Autodesk Inventor part; units mm, degrees
ref_plane "Arbeitsebene1" through (114.85, 0, 0) normal (1, 0, 0) x (0, 1, 0)
ref_plane "Arbeitsebene2" through (25.15, 0, 0) normal (1, 0, 0) x (0, 1, 0)
ref_plane "YZ Plane" through (0, 0, 0) normal (1, 0, 0) x (0, 1, 0)
sketch "Skizze1" plane through (0, 0, 0) normal (1, 0, 0) x (0, 1, 0)
  circle A0 centre (0, 0) radius 5
  dimension "d0" = 10
extrude "Extrusion1" add sketch "Skizze1" along normal blind 140
sketch "Skizze2" plane through (0, 0, 0) normal (-1, 0, 0) x (0, 0, 1)
  point P0 (0, 0)
  point P1 (0, 0)
hole "Bohrung1" at (0, 0, 0) direction (1, 0, 0) diameter 4.134 depth 14.2 tip angle 118
sketch "Skizze3" plane through (140, 0, 0) normal (1, 0, 0) x (0, 0, -1)
  point P0 (0, 0)
  point P1 (0, 0)
hole "Bohrung2" at (140, 0, 0) direction (-1, 0, 0) diameter 4.134 depth 14.2 tip angle 118
sketch "Skizze4" plane through (0, 0, 0) normal (0, 1, 0) x (-1, 0, 0)
  line L0 (0, 0) -> (-70, 0)
  line L1 (-70, 0) -> (-140, 0)
  line L2 (-140, -2.067) -> (-140, 2.067)
  line L3 (-70, 0) -> (-114.85, 0)
  line L4 (-70, 0) -> (-25.15, 0)
  dimension "d17" = 70
  dimension "d18" = 70
  dimension "d19" = 44.85
  dimension "d23" = 44.85
ref_plane "Arbeitsebene1" through (114.85, 0, 0) normal (1, 0, 0) x (0, 1, 0)
sketch "Skizze5" plane through (114.85, 0, 0) normal (1, 0, 0) x (0, 1, 0)
  circle A0 centre (0, 0) radius 5
  circle A1 centre (0, 0) radius 4
  dimension "d20" = 8
extrude "Extrusion2" cut sketch "Skizze5" along normal blind 0.9
ref_plane "Arbeitsebene2" through (25.15, 0, 0) normal (1, 0, 0) x (0, 1, 0)
sketch "Skizze6" plane through (25.15, 0, 0) normal (1, 0, 0) x (0, 1, 0)
  circle A0 centre (0, 0) radius 5
  circle A1 centre (0, 0) radius 4
  dimension "d24" = 8
extrude "Extrusion3" cut sketch "Skizze6" against normal blind 0.9
properties part number "Auspressrolle"
Can you work these out from the model? Positions are in its coordinate system, mm. A direction names the side the tool comes from. Coordinates: 2 decimals unless noted, no trailing zeros. Loops run counter-clockwise (first coordinate to the right, second up) from the corner with the lowest first, then second, coordinate; pieces in that order, holes last. Notation, with made-up numbers: (67.5, 87) -> (72.5, 87) arc R27 ccw to (72.5, 112) -> close; hole circle Ø9 at (-27, 60). An arc over 180 degrees is marked (long way). Answer as a JSON object with one key per item and string values.
1) For faces 1 (the face through (115.294, -0.867, 3.905)), 2 (the face through (7.2, 1.26, -1.64)), 3 (the face through (127.71, -1.08, 4.88)), which set-ups out of +Z, -Z, +X, -X, +Y, -Y let a thin tool reach every point of the face, with its end or its side?
Results:
{"face 1": "none", "face 2": "-X", "face 3": "+X, -X"}
2) Imagine slicing it at A-A (x = 35). Please give me the cut outline in (y, z).
Results:
{"outline": "circle Ø10 at (0, 0)"}
3) For P1, Ø3, axis at x = 97.5, y = 2.5, coming from the +Z side; P2, Ø2.5, axis at y = 0, z = 0, coming from the -X side; P3, Ø3, axis at x = 75.5, z = 2, coming from the +Y side, each with a flat end and sliding along its axis, tell me the tip position at first contact or that it passes through.
Results:
{"P1": "stops at z = 4.9", "P2": "stops at x = 14.69", "P3": "stops at y = 4.97"}
4) Thinking about a two-plate mould opening in Y: for faces 4 (the face through (0, 2, -1)), 5 (the face through (132.8, 1.26, 1.64)), 6 (the face through (24.706, -0.867, -3.905)), which applies, pulls with the +Y half, pulls with the -Y half, needs draft (parallel to the pull), parting line crosses it, or undercut?
Results:
{"face 4": "needs draft", "face 5": "undercut", "face 6": "parting line crosses it"}
5) If I drill on line 1 (X direction, y = 4, z = 2); line 2 (Z direction, x = 134.5, y = 0); line 3 (Z direction, x = 21, y = -3), over which ranges is the centre line in solid material (lowest first)?
Results:
{"line 1": "x = 0 to 24.25, 25.15 to 114.85, 115.75 to 140", "line 2": "z = -5 to -2.07, 2.07 to 5", "line 3": "z = -4 to 4"}
